Work out the finished part from the listing and answer in its coordinate system (mm). Face numbers are marked on the shaded views. A direction names the side the tool comes from. Give positions to 0.01 mm unless a question says otherwise; leave off trailing zeros. Loops run counter-clockwise (first coordinate to the right, second up) from the corner with the lowest first, then second, coordinate; pieces in that order, holes last. Notation, with made-up numbers: M -28,44 L -1,44 A21 ccw -1,67 Z; hole C 19.5,45.25 d2. An arc over 180 degrees is marked long. Write item = value, one per line. Start each with the question number.
1. For the marked faces 4 and 5, determine the directions among +Z, -Z, +X, -X, +Y, -Y from which every point of the face is accessible in a straight line to the end or side of a thin tool.
2. Section C-C on x = 0 is taken. Determine the outline of the cut face in (y, z).
3. The mould has two halves that part along Z. Classify the marked faces 1, 2 and 3: released by +Z, released by -Z, zero draft, split by the parting line, or undercut.
4. Consider L1, parallel to Z at x = 0, y = 24; L2, parallel to Y at x = 6, z = -19.5; L3, parallel to X at y = 1.25, z = -9.75. Determine where each line is inside the solid, lowest interval first. Write a range as [from, to].
5. Section B-B on z = -11.5 is taken. Determine the outline of the cut face in (x, y).
6. A flat-ended cylindrical pin translates along its axis: pin 1 Ø0.9 at (x, z) = (0, -22.5) entering from +Y. Find the tip coordinate at first contact, or state that the pin passes through.
7. Section A-A on x = 4.25 is taken. Determine the outline of the cut face in (y, z), plus the area to 3 significant figures.
8. Section D-D on y = 21.25 is taken. Determine the outline of the cut face in (x, z).
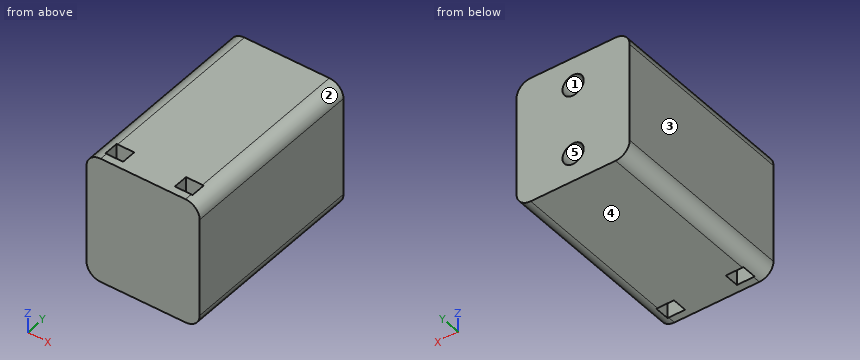
Autodesk Inventor part; units mm, degrees
ref_plane "YZ Plane" through (0, 0, 0) normal (1, 0, 0) x (0, 1, 0)
ref_plane "XZ Plane" through (0, 0, 0) normal (0, 1, 0) x (-1, 0, 0)
ref_plane "XY Plane" through (0, 0, 0) normal (0, 0, 1) x (1, 0, 0)
sketch "Sketch1" plane through (0, 0, 0) normal (0, 1, 0) x (-1, 0, 0)
  circle A0 centre (0, -12.557) radius 1.5
  circle A1 centre (0, -22.557) radius 1.5
  arc A2 (-14.605, -9.6379) -> (-15.8103, -6.9952) centre (-18.105, -9.6379) ccw
  line L0 (-14.605, -29.4809) -> (-14.605, -9.6379)
  line L1 (13.605, -29.4809) -> (-14.605, -29.4809)
  line L2 (13.605, -12.0588) -> (13.605, -29.4809)
  arc A3 (14.5665, -9.2788) -> (13.605, -12.0588) centre (18.105, -12.0588) ccw
  line L3 (0, -22.557) -> (0, -12.557)
  line L4 (-8, -8.557) -> (8, -8.557)
  line L5 (8, -8.557) -> (8, -26.557)
  line L6 (8, -26.557) -> (-8, -26.557)
  line L7 (-8, -26.557) -> (-8, -8.557)
  line L8 (-8, -8.557) -> (8, -26.557) construction
  line L9 (8, -8.557) -> (-8, -26.557) construction
  point P0 (0, -17.557)
  dimension "d0" = 3
  dimension "d1" = 3
  dimension "d2" = 10
  dimension "d3" = 16
  dimension "d4" = 18
extrude "Extrusion1" add sketch "Sketch1" along normal blind 27
extrude "Extrusion2" add sketch "Sketch1" along normal blind 17 contours A0 | A1
fillet "Fillet1" radius 2 4 edges at (-8, 13.5, -8.557) (8, 13.5, -8.557) (-8, 13.5, -26.557) (8, 13.5, -26.557)
sketch "Sketch2" plane through (-6, 0, -8.557) normal (0, 0, 1) x (1, 0, 0)
  line L0 (-0.15, 3.1878) -> (2.35, 3.1878)
  line L1 (2.35, 3.1878) -> (2.35, 1.0878)
  line L2 (2.35, 1.0878) -> (-0.15, 1.0878)
  line L3 (-0.15, 1.0878) -> (-0.15, 3.1878)
  line L4 (-0.15, 3.1878) -> (2.35, 1.0878) construction
  line L5 (2.35, 3.1878) -> (-0.15, 1.0878) construction
  line L6 (9.6689, 3.1878) -> (12.1689, 3.1878)
  line L7 (12.1689, 3.1878) -> (12.1689, 1.0878)
  line L8 (12.1689, 1.0878) -> (9.6689, 1.0878)
  line L9 (9.6689, 1.0878) -> (9.6689, 3.1878)
  line L10 (9.6689, 3.1878) -> (12.1689, 1.0878) construction
  line L11 (12.1689, 3.1878) -> (9.6689, 1.0878) construction
  line L12 (-0.15, 2.1378) -> (12.15, 2.1378) construction
  line L13 (6, 0) -> (6, 2.1378)
  point P0 (1.1, 2.1378)
  point P1 (10.9189, 2.1378)
  point P2 (12.1689, 2.1378)
  dimension "d10" = 2.5
  dimension "d11" = 2.1
  dimension "d12" = 2.5
  dimension "d13" = 2.1
  dimension "d14" = 12.3
extrude "Extrusion3" cut sketch "Sketch2" against normal blind 19.5
properties part number "IR Headtracker riser"
Verdict:
q1.face_4 = -Z, +X, -X, +Y, -Y
q1.face_5 = +Y
q2.outline = M 0,-26.56 L 27,-26.56 L 27,-24.06 L 17,-24.06 L 17,-21.06 L 27,-21.06 L 27,-14.06 L 17,-14.06 L 17,-11.06 L 27,-11.06 L 27,-8.56 L 0,-8.56 Z
q3.face_1 = undercut
q3.face_2 = released by +Z
q3.face_3 = zero draft
q4.L1 = [-26.56, -24.06], [-21.06, -14.06], [-11.06, -8.56]
q4.L2 = [0, 1.09], [3.19, 27]
q4.L3 = [-7.83, -6.15], [-3.65, 3.67], [6.17, 7.83]
q5.outline = M -8,0 L 8,0 L 8,27 L 1.06,27 L 1.06,17 L -1.06,17 L -1.06,27 L -8,27 Z; hole M -6.15,1.09 L -3.65,1.09 L -3.65,3.19 L -6.15,3.19 Z; hole M 3.67,1.09 L 6.17,1.09 L 6.17,3.19 L 3.67,3.19 Z
q6.pin_1 = 17
q7.outline = M 0,-26.56 L 1.09,-26.56 L 1.09,-8.56 L 0,-8.56 Z; M 3.19,-26.56 L 27,-26.56 L 27,-8.56 L 3.19,-8.56 Z
q7.area = 448 mm2
q8.outline = M -8,-24.56 A2 ccw -6,-26.56 L 6,-26.56 A2 ccw 8,-24.56 L 8,-10.56 A2 ccw 6,-8.56 L -6,-8.56 A2 ccw -8,-10.56 Z; hole C 0,-22.56 d3; hole C 0,-12.56 d3
